Source: CAD feature listing. Evaluate the final solid. Frame: model axes, mm. Give positions to 0.01 mm unless a question says otherwise; leave off trailing zeros. Order: outer loops, then holes, each group sorted by start corner. A loop starts at its lowest first (then second) coordinate and runs counter-clockwise, first axis right, second up. Notation, with made-up numbers: M -34.5,89 L 10.5,89 A17 ccw 10.5,114 Z; hole C 39,84.5 d8. An arc over 180 degrees is marked long. Return JSON: item names as keys, results as strings.
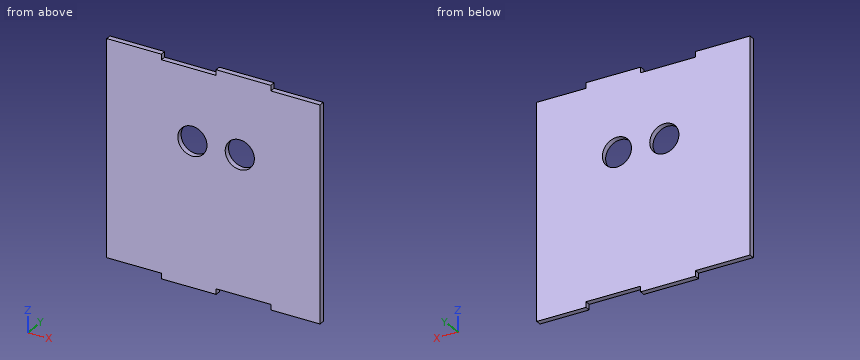
from build123d import *

# Parameters (mm, degrees)
F0_R     = 8
F1_DEPTH = 1.5


# Not quite as in the source:
# - a feature names something its author has since deleted; it is built from what else it names


with BuildPart() as f1:
    # F0 (on Front) → F1 (new body, symmetric)
    with BuildSketch(Plane.XZ):
        Polygon((-30, -2.9994321861), (0, -2.9994321861), (0, 0), (30, 0), (30, -2.9994321861), (57, -2.9994321861), (57, 114.0005678139), (30, 114.0005678139), (30, 117.0005678139), (0, 117.0005678139), (0, 114.0005678139), (-30, 114.0005678139), (-30, 117.0005678139), (-60, 117.0005678139), (-60, 0), (-30, 0), align=None)
        with Locations((-13, 75.2281695604)):
            Circle(F0_R, mode=Mode.SUBTRACT)
        with Locations((13, 75.2218647463)):
            Circle(F0_R, mode=Mode.SUBTRACT)
    extrude(amount=F1_DEPTH, both=True)


solid = f1.part
1. First-contact query: pin 1 (0.9 mm diameter, centred on x = -20.5, y = 0, fed in from +Z); pin 2 (1.5 mm diameter, centred on y = 0, z = 116, fed in from +X); pin 3 (0.9 mm diameter, centred on y = -0.5, z = -1.5, fed in from -X). Flat tips, straight axial feed; report the tip coordinate or a pass-through.
Evaluation:
{"pin 1": "stops at z = 114", "pin 2": "stops at x = 30", "pin 3": "stops at x = -30"}
2. Section query B-B (y = 0.75). Return loops of the section in (x, z).
Evaluation:
{"outline": "M -60,0 L -30,0 L -30,-3 L 0,-3 L 0,0 L 30,0 L 30,-3 L 57,-3 L 57,114 L 30,114 L 30,117 L 0,117 L 0,114 L -30,114 L -30,117 L -60,117 Z; hole C -13,75.23 d16; hole C 13,75.22 d16"}
3. Section query C-C (x = -13). Return loops of the section in (y, z), then the cut area to 3 significant figures.
Evaluation:
{"outline": "M -1.5,-3 L 1.5,-3 L 1.5,67.23 L -1.5,67.23 Z; M -1.5,83.23 L 1.5,83.23 L 1.5,114 L -1.5,114 Z", "area": "303 mm^2"}
4. Section query D-D (x = -35.5). Return loops of the section in (y, z).
Evaluation:
{"outline": "M -1.5,0 L 1.5,0 L 1.5,117 L -1.5,117 Z"}
5. Section query A-A (x = 13). Return loops of the section in (y, z).
Evaluation:
{"outline": "M -1.5,0 L 1.5,0 L 1.5,67.22 L -1.5,67.22 Z; M -1.5,83.22 L 1.5,83.22 L 1.5,117 L -1.5,117 Z"}
6. Ray query, probe 1 along X at (y, z) = (-0.1, 75.5); probe 2 along Z at (x, y) = (-13, -0.05); probe 3 along Z at (x, y) = (50.5, -0.7). Return the intervals inside material, ascending.
Evaluation:
{"probe 1": "x = -60 to -21, -5 to 5, 21 to 57", "probe 2": "z = -3 to 67.23, 83.23 to 114", "probe 3": "z = -3 to 114"}
